from build123d import *

# Parameters (mm, degrees)
BOSS_EXTRUDE1_DEPTH = 76.2
CHAMFER1_SIZE       = 0.254


with BuildPart() as part:
    # Sketch1 → Boss-Extrude1 (new body)
    with BuildSketch(Plane(origin=(0, 0, 0), x_dir=(1, 0, 0), z_dir=(0, 1, 0))):
        with BuildLine():
            ThreePointArc((2.091397583, 1.203588447), (0, 2.413), (-2.091397583, 1.203588447))
            Line((-2.091397583, 1.203588447), (2.091397583, 1.203588447))
        make_face()
        with BuildLine():
            Line((2.091397583, 1.203588447), (-2.091397583, 1.203588447))
            ThreePointArc((-2.091397583, 1.203588447), (-0.622907149, -2.33121335), (2.413, 0))
            ThreePointArc((2.413, 0), (2.33121335, 0.622907149), (2.091397583, 1.203588447))
        make_face()
    extrude(amount=BOSS_EXTRUDE1_DEPTH)

    # Chamfer1
    chamfer1_edges = [part.edges().sort_by_distance(p)[0] for p in [
        (-2.091397583, 0, 1.203588447),
        (-2.091397583, 76.2, 1.203588447),
    ]]
    chamfer(chamfer1_edges, length=CHAMFER1_SIZE)


solid = part.part
CAD build for the part. Positions are in the model's coordinates, mm. Give positions to 0.01 mm unless a question says otherwise; leave off trailing zeros. Write each loop counter-clockwise with the first axis right and the second up, starting at its lowest first coordinate (ties: lowest second). Pieces come first, ordered by that corner, then holes. Notation, with made-up numbers: (-13.75, -9.75) -> (-0.75, -9.75) arc R13 cw to (-0.75, 5.25) -> close; hole circle Ø8 at (-6.75, 4). An arc over 180 degrees is marked (long way). Return JSON: item names as keys, results as strings.
Item 1: Drop flat-ended pins along their axis: pin 1 (1 mm diameter, centred on y = 10.5, z = -1.5, fed in from +X); pin 2 (1.5 mm diameter, centred on x = -1, y = 29.5, fed in from +Z). Give the stop position or say it passes through.
Answer below:
{"pin 1": "stops at x = 2.2", "pin 2": "stops at z = 2.4"}
Item 2: Band-saw the part on A-A (y = 57). List the corners of the cut face in (x, z), then the cut area to 3 significant figures.
Answer below:
{"outline": "circle Ø4.83 at (0, 0)", "area": "18.3 mm2"}
Item 3: Drill centre lines: probe 1 along Z at (x, y) = (0.2, 54.5); probe 2 along Z at (x, y) = (-1.1, 57). Where is each one in solid material? Low to high.
Answer below:
{"probe 1": "z = -2.4 to 2.4", "probe 2": "z = -2.15 to 2.15"}
